Part print with two shaded views. Sizes in mm from the minimum x, y, z corner. A direction names the side the tool comes from. Round coordinates to 2 decimals unless told otherwise and drop trailing zeros. Loops run counter-clockwise (first coordinate to the right, second up) from the corner with the lowest first, then second, coordinate; pieces in that order, holes last. Notation, with made-up numbers: (85.25, -4.75) - (127.25, -4.75) arc R24 ccw to (127.25, 21.25) - close; hole circle Ø10 at (39, -12). An arc over 180 degrees is marked (long way). Write each question's results on one line, items separated by ' | '. Start each with the question number.
(1) Cut at B-B, the plane x = 18. List the corners of the cut face in (y, z).
(2) Cut at C-C, the plane y = 12.5. List the corners of the cut face in (x, z) (1 decimal).
(3) Mould opens along Z. For the marked faces 1, 2, 3 and 4 say: released by +Z, released by -Z, zero draft, split by the parting line, or undercut.
(4) Cut at A-A, the plane z = 15. Give the number of separate pieces and of enclosed holes in the cut face.
(5) Flat gauge pin, fed straight in: P1, Ø1, axis at y = 4, z = 37, coming from the -X side. Where does the tip first touch, or does it go through?
(6) Cut at D-D, the plane x = 24. List the corners of the cut face in (y, z), then the cut area to 3 significant figures.
(7) Drill centre lines: L1, parallel to X at y = 3.5, z = 15; L2, parallel to X at y = 7.25, z = 15 (1 decimal); L3, parallel to Z at x = 38, y = 3.2. Where is each one in solid material? Low to high.
(8) Tool access for the marked faces 5 and 6: list every direction of +Z, -Z, +X, -X, +Y, -Y with a clear straight run to the whole face (end or side of a thin tool).
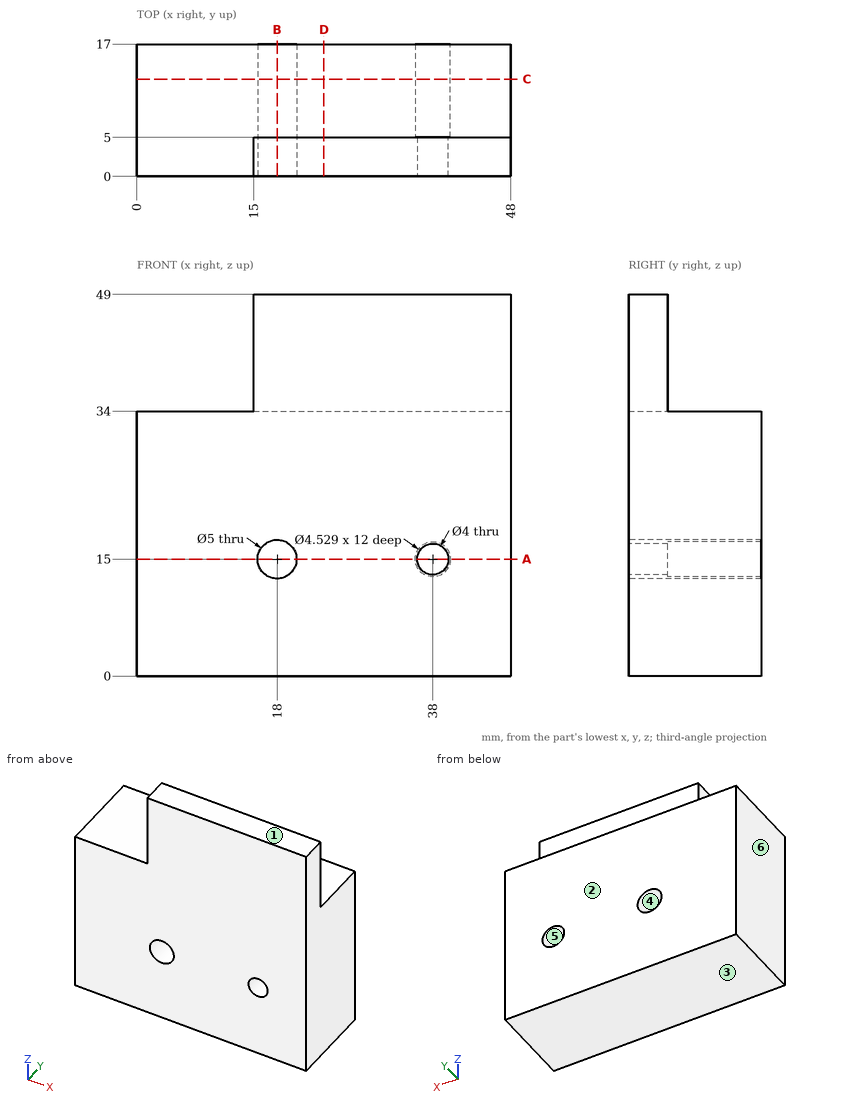
A:
1) outline: (0, 0) - (17, 0) - (17, 12.5) - (0, 12.5) - close; (0, 17.5) - (17, 17.5) - (17, 34) - (5, 34) - (5, 49) - (0, 49) - close
2) outline: (0, 0) - (48, 0) - (48, 34) - (0, 34) - close; hole circle Ø5 at (18, 15); hole circle Ø4.5 at (38, 15)
3) face 1: released by +Z | face 2: zero draft | face 3: released by -Z | face 4: undercut
4) separate pieces: 3 | enclosed holes: 0
5) P1: x = 15
6) outline: (0, 0) - (17, 0) - (17, 34) - (5, 34) - (5, 49) - (0, 49) - close | area: 653 mm2
7) L1: 0 to 15.5, 20.5 to 36, 40 to 48 | L2: 0 to 15.5, 20.5 to 35.7, 40.3 to 48 | L3: 0 to 13, 17 to 49
8) face 5: +Y | face 6: +Z, -Z, -X, +Y, -Y
